Answer from the drawing. Dimensions are ordinates in mm from the lowest x, y and z of the part. Coordinates: 2 decimals unless noted, no trailing zeros. Write each loop counter-clockwise with the first axis right and the second up, starting at its lowest first coordinate (ties: lowest second). Pieces come first, ordered by that corner, then holes. Notation, with made-up numbers: (-35, 82.5) - (6, 82.5) arc R23 cw to (6, 92.5) - close; hole circle Ø7 at (79.5, -21). An arc over 180 degrees is marked (long way). Use a Markdown table: item, result.
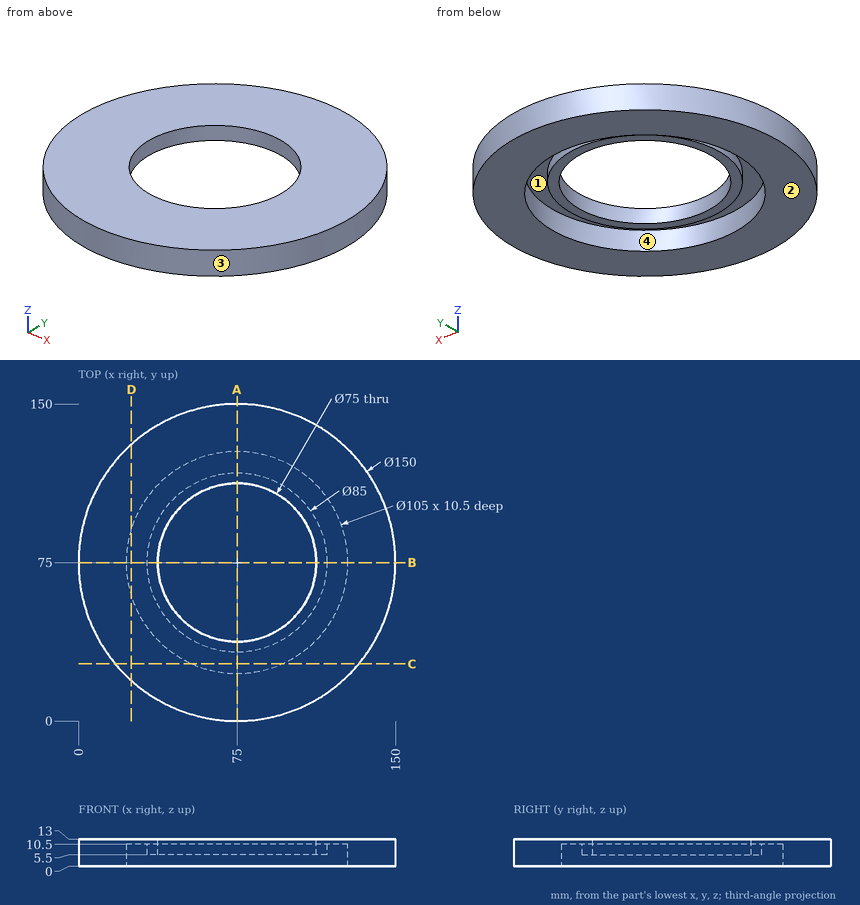
(1) A cutting plane is placed at C-C, the plane y = 27. Write down the section's boundary in (x, z).
Report:
| item | result |
|---|---|
| outline | (17.37, 0) - (53.73, 0) - (53.73, 10.5) - (96.27, 10.5) - (96.27, 0) - (132.63, 0) - (132.63, 13) - (17.37, 13) - close |
(2) The mould has two halves that part along Y. Classify the marked faces 1, 2, 3 and 4: pulls with the +Y half, pulls with the -Y half, needs draft (parallel to the pull), parting line crosses it, or undercut.
Report:
| item | result |
|---|---|
| face 1 | undercut |
| face 2 | needs draft |
| face 3 | parting line crosses it |
| face 4 | undercut |
(3) Each of these flat-tipped pins is pushed along its axis until it touches: P1, Ø1, axis at y = 58.5, z = 8, coming from the -X side; P2, Ø3, axis at y = 35, z = 10.5, coming from the +X side; P3, Ø4, axis at y = 84.5, z = 1.5, coming from the +X side. Where does it stop, or does it pass through?
Report:
| item | result |
|---|---|
| P1 | stops at x = 1.73 |
| P2 | stops at x = 139.36 |
| P3 | stops at x = 149.62 |
(4) A cutting plane is placed at A-A, the plane x = 75. Write down the section's boundary in (y, z).
Report:
| item | result |
|---|---|
| outline | (0, 0) - (22.5, 0) - (22.5, 10.5) - (32.5, 10.5) - (32.5, 5.5) - (37.5, 5.5) - (37.5, 13) - (0, 13) - close; (112.5, 5.5) - (117.5, 5.5) - (117.5, 10.5) - (127.5, 10.5) - (127.5, 0) - (150, 0) - (150, 13) - (112.5, 13) - close |
(5) Straight lines are drawn through the part: L1, parallel to Y at x = 75, z = 6; L2, parallel to Y at x = 95, z = 5.75; L3, parallel to Z at x = 61.5, y = 124.5. For each, find the intervals that lie inside material, in ascending order.
Report:
| item | result |
|---|---|
| L1 | y = 0 to 22.5, 32.5 to 37.5, 112.5 to 117.5, 127.5 to 150 |
| L2 | y = 2.72 to 26.46, 37.5 to 43.28, 106.72 to 112.5, 123.54 to 147.28 |
| L3 | z = 10.5 to 13 |
(6) A cutting plane is placed at D-D, the plane x = 25. Write down the section's boundary in (y, z).
Report:
| item | result |
|---|---|
| outline | (19.1, 0) - (58.99, 0) - (58.99, 10.5) - (91.01, 10.5) - (91.01, 0) - (130.9, 0) - (130.9, 13) - (19.1, 13) - close |
